Check sheet for the modelled part. Datum: model origin and axes. Units: mm. Give positions to 0.01 mm unless a question says otherwise; leave off trailing zeros. Loops run counter-clockwise (first coordinate to the right, second up) from the corner with the lowest first, then second, coordinate; pieces in that order, holes last. Notation, with made-up numbers: M -28.75,-5.5 L 30.25,-5.5 A4 ccw 30.25,1.5 Z; hole C 4.5,-13 d5. An arc over 180 degrees is marked long. Write each question's results on one line, items separated by ' | '. Start each with the question number.
1. Draft check along X on faces 1 (the cylindrical face through (27, 1.6, 5.5)), 2 (the flat face through (-1, 0, 0)), 3 (the flat face through (50, 0, 4)), 4 (the conical face through (-33.143, 1.638, 2.854)). Enter one of: pulls with the +X half, pulls with the -X half, needs draft (parallel to the pull), parting line crosses it, or undercut.
2. Go/stop test with a flat-tipped pin: pin 1 (7 mm diameter, centred on x = 30, y = 1.5, fed in from -Z). Record where the tip stops, or that it passes through.
3. Sectioned sample at C-C on x = 30. Record the cut outline in (y, z), and give its area (3 significant figures).
4. Material ranges on line 1 along X through (y, z) = (1.5, 6.35); line 2 along Y through (x, z) = (30, 7); line 3 along Z through (x, y) = (33, 1), recorded low to high.
5. Sectioned sample at B-B on z = 4. Record the cut outline in (x, y), and give its area (3 significant figures).
6. Sectioned sample at A-A on y = 1.5. Record the cut outline in (x, z), and give its area (3 significant figures).
```python
from build123d import *

# Parameters (mm, degrees)
SKETCH1_W                                           = 100
SKETCH1_H                                           = 28
BOSS_EXTRUDE1_DEPTH                                 = 8
CSK_FOR_M6_COUNTERSUNK_FLAT_HEAD_SCREW1_D           = 6
CSK_FOR_M6_COUNTERSUNK_FLAT_HEAD_SCREW1_CSINK_D     = 12
CSK_FOR_M6_COUNTERSUNK_FLAT_HEAD_SCREW1_CSINK_ANGLE = 90


with BuildPart() as part:
    # Sketch1 → Boss-Extrude1 (new body)
    with BuildSketch(Plane.XY):
        Rectangle(SKETCH1_W, SKETCH1_H)
    extrude(amount=BOSS_EXTRUDE1_DEPTH)

    # CSK for M6 Countersunk Flat Head Screw1 (through all)
    with Locations(Plane(origin=(0, 0, 0), x_dir=(-1, 0, 0), z_dir=(0, 0, -1))):
        with Locations((30, 1.5), (-30, 1.5)):
            CounterSinkHole(CSK_FOR_M6_COUNTERSUNK_FLAT_HEAD_SCREW1_D / 2, CSK_FOR_M6_COUNTERSUNK_FLAT_HEAD_SCREW1_CSINK_D / 2, counter_sink_angle=CSK_FOR_M6_COUNTERSUNK_FLAT_HEAD_SCREW1_CSINK_ANGLE)


solid = part.part
```
Output values:
1) face 1: undercut | face 2: needs draft | face 3: pulls with the +X half | face 4: undercut
2) pin 1: z = 2.5
3) outline: M -14,0 L -4.5,0 L -1.5,3 L -1.5,8 L -14,8 Z; M 4.5,3 L 7.5,0 L 14,0 L 14,8 L 4.5,8 Z | area: 167 mm2
4) line 1: -50 to -33, -27 to 27, 33 to 50 | line 2: -14 to -1.5, 4.5 to 14 | line 3: 2.96 to 8
5) outline: M -50,-14 L 50,-14 L 50,14 L -50,14 Z; hole C -30,1.5 d6; hole C 30,1.5 d6 | area: 2,740 mm2
6) outline: M -50,0 L -36,0 L -33,3 L -33,8 L -50,8 Z; M -27,3 L -24,0 L 24,0 L 27,3 L 27,8 L -27,8 Z; M 33,3 L 36,0 L 50,0 L 50,8 L 33,8 Z | area: 686 mm2
